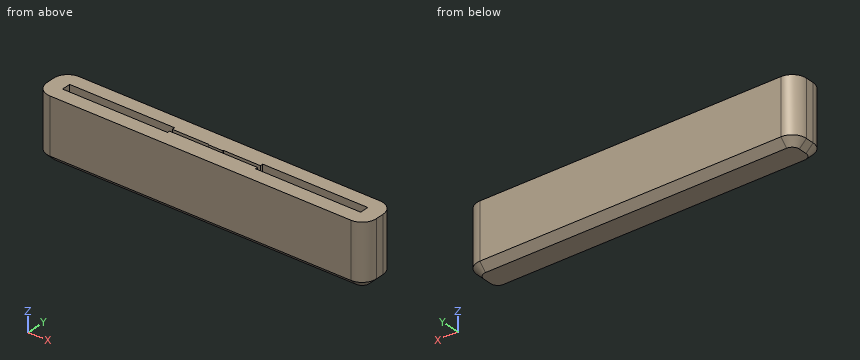
from build123d import *

# Parameters (mm, degrees)
F0_W     = 46.4
F0_H     = 5.2
F0_W_2   = 14.8002340496
F0_H_2   = 0.4131594501
F0_H_3   = 0.3522689282
F1_DEPTH = 2
F2_DEPTH = 6.8
F3_R     = 2
F4_SIZE  = 1
F5_W     = 2
F5_H     = 0.1
F6_DEPTH = 2


with BuildPart() as f1:
    # F0 (on Top) → F1 (new body)
    with BuildSketch(Plane.XY):
        with Locations((0, -2.6)):
            Rectangle(F0_W, F0_H)
        Polygon((-21, -2.85), (-21, -2.35), (-21, -1.9368405499), (-6.1997659504, -1.9368405499), (-6.1997659504, -2.35), (0, -2.35), (6.1997659504, -2.35), (6.1997659504, -1.9368405499), (21, -1.9368405499), (21, -2.35), (21, -2.85), (21, -3.2022689282), (6.1997659504, -3.2022689282), (6.1997659504, -2.85), (0, -2.85), (-6.1997659504, -2.85), (-6.1997659504, -3.2022689282), (-21, -3.2022689282), align=None, mode=Mode.SUBTRACT)
        Polygon((-6.1997659504, -2.35), (-21, -2.35), (-21, -2.85), (-6.1997659504, -2.85), (0, -2.85), (6.1997659504, -2.85), (21, -2.85), (21, -2.35), (6.1997659504, -2.35), (0, -2.35), align=None)
        with Locations((-13.5998829752, -2.143420275)):
            Rectangle(F0_W_2, F0_H_2)
        with Locations((13.5998829752, -2.143420275)):
            Rectangle(F0_W_2, F0_H_2)
        with Locations((-13.5998829752, -3.0261344641)):
            Rectangle(F0_W_2, F0_H_3)
        with Locations((13.5998829752, -3.0261344641)):
            Rectangle(F0_W_2, F0_H_3)
    extrude(amount=-F1_DEPTH)

    # F0 (on Top) → F2 (join)
    with BuildSketch(Plane.XY):
        with Locations((0, -2.6)):
            Rectangle(F0_W, F0_H)
        Polygon((-21, -2.85), (-21, -2.35), (-21, -1.9368405499), (-6.1997659504, -1.9368405499), (-6.1997659504, -2.35), (0, -2.35), (6.1997659504, -2.35), (6.1997659504, -1.9368405499), (21, -1.9368405499), (21, -2.35), (21, -2.85), (21, -3.2022689282), (6.1997659504, -3.2022689282), (6.1997659504, -2.85), (0, -2.85), (-6.1997659504, -2.85), (-6.1997659504, -3.2022689282), (-21, -3.2022689282), align=None, mode=Mode.SUBTRACT)
    extrude(amount=F2_DEPTH)

    # F3
    f3_edges = [f1.edges().sort_by_distance(p)[0] for p in [
        (23.2, -5.2, 2.4),
        (23.2, 0, 2.4),
        (-23.2, -5.2, 2.4),
        (-23.2, 0, 2.4),
    ]]
    fillet(f3_edges, radius=F3_R)

    # F4
    f4_edges = [f1.edges().sort_by_distance(p)[0] for p in [
        (0, 0, -2),
        (22.614214, -0.585786, -2),
        (-22.614214, -0.585786, -2),
        (23.2, -2.6, -2),
        (-23.2, -2.6, -2),
        (22.614214, -4.614214, -2),
        (-22.614214, -4.614214, -2),
        (0, -5.2, -2),
    ]]
    chamfer(f4_edges, length=F4_SIZE)

    # F5 (on face) → F6 (join)
    with BuildSketch(Plane.XY.offset(6.8)):
        with Locations((0, -2.4)):
            Rectangle(F5_W, F5_H)
    extrude(amount=-F6_DEPTH)


solid = f1.part
The model under review builds one solid part; all positions refer to its coordinate system, in mm. Coordinates: 2 decimals unless noted, no trailing zeros. Loops run counter-clockwise (first coordinate to the right, second up) from the corner with the lowest first, then second, coordinate; pieces in that order, holes last. Notation, with made-up numbers: (-7.75, 26) -> (13.25, 26) arc R17 ccw to (13.25, 45) -> close; hole circle Ø10 at (70, 16). An arc over 180 degrees is marked (long way). Use a Markdown table: item, result. Add a question column.
1. Add section A-A on z = 5.75. Write out the cut boundary in (x, y), plus the area to 3 significant figures.
2. To check wall thickness, follow line 1 (X direction, y = -2.9, z = 3); line 2 (Y direction, x = 19.5, z = 5.5); line 3 (Y direction, x = -1, z = 2). State the ranges of each line that lie inside material, in increasing order.
3. Add section B-B on x = 2. Write out the cut boundary in (y, z), plus the area to 3 significant figures.
4. Add section D-D on x = 11.5. Write out the cut boundary in (y, z), plus the area to 3 significant figures.
5. Add section C-C on z = 2.5. Write out the cut boundary in (x, y).
Returned:
| question | item | result |
|---|---|---|
| 1 | outline | (-23.2, -3.2) arc R2 ccw to (-21.2, -5.2) -> (21.2, -5.2) arc R2 ccw to (23.2, -3.2) -> (23.2, -2) arc R2 ccw to (21.2, 0) -> (-21.2, 0) arc R2 ccw to (-23.2, -2) -> close; hole (-21, -3.2) -> (-6.2, -3.2) -> (-6.2, -2.85) -> (6.2, -2.85) -> (6.2, -3.2) -> (21, -3.2) -> (21, -1.94) -> (6.2, -1.94) -> (6.2, -2.35) -> (1, -2.35) -> (1, -2.45) -> (-1, -2.45) -> (-1, -2.35) -> (-6.2, -2.35) -> (-6.2, -1.94) -> (-21, -1.94) -> close |
| 1 | area | 194 mm² |
| 2 | line 1 | x = -23.2 to -21, -6.2 to 6.2, 21 to 23.2 |
| 2 | line 2 | y = -5.2 to -3.2, -1.94 to 0 |
| 2 | line 3 | y = -5.2 to -2.85, -2.35 to 0 |
| 3 | outline | (-5.2, -1) -> (-4.2, -2) -> (-1, -2) -> (0, -1) -> (0, 6.8) -> (-2.35, 6.8) -> (-2.35, 0) -> (-2.85, 0) -> (-2.85, 6.8) -> (-5.2, 6.8) -> close |
| 3 | area | 41.4 mm² |
| 4 | outline | (-5.2, -1) -> (-4.2, -2) -> (-1, -2) -> (0, -1) -> (0, 6.8) -> (-1.94, 6.8) -> (-1.94, 0) -> (-3.2, 0) -> (-3.2, 6.8) -> (-5.2, 6.8) -> close |
| 4 | area | 36.2 mm² |
| 5 | outline | (-23.2, -3.2) arc R2 ccw to (-21.2, -5.2) -> (21.2, -5.2) arc R2 ccw to (23.2, -3.2) -> (23.2, -2) arc R2 ccw to (21.2, 0) -> (-21.2, 0) arc R2 ccw to (-23.2, -2) -> close; hole (-21, -3.2) -> (-6.2, -3.2) -> (-6.2, -2.85) -> (6.2, -2.85) -> (6.2, -3.2) -> (21, -3.2) -> (21, -1.94) -> (6.2, -1.94) -> (6.2, -2.35) -> (-6.2, -2.35) -> (-6.2, -1.94) -> (-21, -1.94) -> close |
